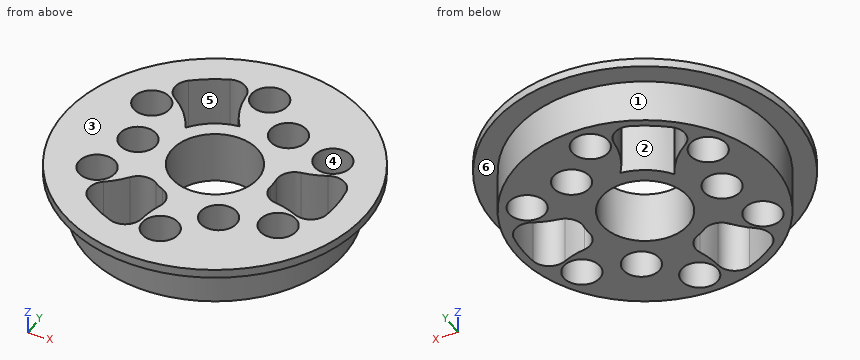
from build123d import *

# Parameters (mm, degrees)
SKETCH_1_R          = 15
SKETCH_1_R_2        = 2.1
EXTRUDE_1_DEPTH     = 6
EXTRUDE_START       = -1
SKETCH_2_R          = 17.5
SKETCH_2_R_2        = 2.1
EXTRUDE_2_DEPTH     = 1
SKETCH_3_R          = 5
CUT_EXTRUDE_1_DEPTH = 10
CUT_EXTRUDE_3_DEPTH = 10
FILLET_1_R          = 2


with BuildPart() as part:
    # 草图1 → 凸台-拉伸1 (new body)
    with BuildSketch(Plane.XY):
        Circle(SKETCH_1_R)
        with Locations((0, 12)):
            Circle(SKETCH_1_R_2, mode=Mode.SUBTRACT)
        with Locations((10.392304845, 6)):
            Circle(SKETCH_1_R_2, mode=Mode.SUBTRACT)
        with Locations((10.392304845, -6)):
            Circle(SKETCH_1_R_2, mode=Mode.SUBTRACT)
        with Locations((0, -12)):
            Circle(SKETCH_1_R_2, mode=Mode.SUBTRACT)
        with Locations((-10.392304845, -6)):
            Circle(SKETCH_1_R_2, mode=Mode.SUBTRACT)
        with Locations((-10.392304845, 6)):
            Circle(SKETCH_1_R_2, mode=Mode.SUBTRACT)
        with Locations((4.425, 7.664324823)):
            Circle(SKETCH_1_R_2, mode=Mode.SUBTRACT)
        with Locations((4.419693866, -7.655134331)):
            Circle(SKETCH_1_R_2, mode=Mode.SUBTRACT)
        with Locations((-8.844693866, 0.009190493)):
            Circle(SKETCH_1_R_2, mode=Mode.SUBTRACT)
    extrude(amount=EXTRUDE_1_DEPTH)

    # 草图2 → 凸台-拉伸2 (add)
    with BuildSketch(Plane.XY.offset(6).offset(EXTRUDE_START)):
        Circle(SKETCH_2_R)
        with Locations((-8.844693866, 0.009190493)):
            Circle(SKETCH_2_R_2, mode=Mode.SUBTRACT)
        with Locations((-10.392304845, -6)):
            Circle(SKETCH_2_R_2, mode=Mode.SUBTRACT)
        with Locations((0, -12)):
            Circle(SKETCH_2_R_2, mode=Mode.SUBTRACT)
        with Locations((4.419693866, -7.655134331)):
            Circle(SKETCH_2_R_2, mode=Mode.SUBTRACT)
        with Locations((10.392304845, -6)):
            Circle(SKETCH_2_R_2, mode=Mode.SUBTRACT)
        with Locations((10.392304845, 6)):
            Circle(SKETCH_2_R_2, mode=Mode.SUBTRACT)
        with Locations((4.425, 7.664324823)):
            Circle(SKETCH_2_R_2, mode=Mode.SUBTRACT)
        with Locations((0, 12)):
            Circle(SKETCH_2_R_2, mode=Mode.SUBTRACT)
        with Locations((-10.392304845, 6)):
            Circle(SKETCH_2_R_2, mode=Mode.SUBTRACT)
    extrude(amount=EXTRUDE_2_DEPTH)

    # 草图3 → 切除-拉伸1 (cut)
    with BuildSketch(Plane.XY.offset(6)):
        Circle(SKETCH_3_R)
    extrude(amount=-CUT_EXTRUDE_1_DEPTH, mode=Mode.SUBTRACT)

    # 草图4 → 切除-拉伸3 (cut)
    with BuildSketch(Plane(origin=(0, 0, 0), x_dir=(-1, 0, 0), z_dir=(0, 0, -1))):
        with BuildLine():
            ThreePointArc((5.465336879, 3.961387736), (7.679309109, 7.001766097), (10.89964539, 8.94470404))
            ThreePointArc((10.89964539, 8.94470404), (7.05, 12.210958193), (2.296518233, 13.91172182))
            ThreePointArc((2.296518233, 13.91172182), (2.224052757, 10.151359821), (0.697993974, 6.713814446))
            ThreePointArc((0.697993974, 6.713814446), (3.375, 5.845671476), (5.465336879, 3.961387736))
        make_face()
        with BuildLine():
            ThreePointArc((2.296518233, -13.91172182), (7.05, -12.210958193), (10.89964539, -8.94470404))
            ThreePointArc((10.89964539, -8.94470404), (7.679309109, -7.001766097), (5.465336879, -3.961387736))
            ThreePointArc((5.465336879, -3.961387736), (3.375, -5.845671476), (0.697993974, -6.713814446))
            ThreePointArc((0.697993974, -6.713814446), (2.224052757, -10.151359821), (2.296518233, -13.91172182))
        make_face()
        with BuildLine():
            ThreePointArc((-6.163330853, 2.75242671), (-9.903361866, 3.149593723), (-13.196163623, 4.96701778))
            ThreePointArc((-13.196163623, 4.96701778), (-14.1, 0), (-13.196163623, -4.96701778))
            ThreePointArc((-13.196163623, -4.96701778), (-9.903361866, -3.149593723), (-6.163330853, -2.75242671))
            ThreePointArc((-6.163330853, -2.75242671), (-6.75, 0), (-6.163330853, 2.75242671))
        make_face()
    extrude(amount=-CUT_EXTRUDE_3_DEPTH, mode=Mode.SUBTRACT)

    # 圆角1
    fillet_1_edges = [part.edges().sort_by_distance(p)[0] for p in [
        (-10.89964539, 8.94470404, 3),
        (-2.296518233, 13.91172182, 3),
        (-2.296518233, -13.91172182, 3),
        (-0.697993974, -6.713814446, 3),
        (-5.465336879, -3.961387736, 3),
        (-10.89964539, -8.94470404, 3),
        (6.163330853, -2.75242671, 3),
        (13.196163623, -4.96701778, 3),
        (13.196163623, 4.96701778, 3),
        (6.163330853, 2.75242671, 3),
    ]]
    fillet(fillet_1_edges, radius=FILLET_1_R)


solid = part.part
Work out the finished part from the listing and answer in its coordinate system (mm). Face numbers are marked on the shaded views. A direction names the side the tool comes from. Round coordinates to 2 decimals unless told otherwise and drop trailing zeros. Order: outer loops, then holes, each group sorted by start corner. A loop starts at its lowest first (then second) coordinate and runs counter-clockwise, first axis right, second up. Notation, with made-up numbers: M 12,41.25 L 53,41.25 A11 cw 53,52.25 Z; hole C 36,86.25 d1. An arc over 180 degrees is marked long. Put each result on its own line as item: value. Start each with the question number.
Q1. Section B-B, the plane y = 6 is taken. Write down the section's boundary in (x, z).
Q2. Flat-ended cylindrical pins translate along their axes: pin 1 (4 mm diameter, centred on x = 0, y = 12, fed in from -Z); pin 2 (1 mm diameter, centred on x = -2, z = 3, fed in from -Y); pin 3 (1.5 mm diameter, centred on x = 11, z = 3, fed in from +Y). Find the tip coordinate at first contact, or state that the pin passes through.
Q3. Straight lines are drawn through the part: L1, parallel to Y at x = 0, z = 1.95; L2, parallel to Y at x = -11, z = 4; L3, parallel to X at y = 1.5, z = 3.25. For each, find the intervals that lie inside material, in ascending order. Write a range as [from, to].
Q4. A tool of negligible diameter and unlimited length cuts with its end or side. For the marked faces 5 and 6, from which of +Z, -Z, +X, -X, +Y, -Y can it reach the whole face along a straight path? Write none if from no direction.
Q5. Section D-D, the plane y = -12 is taken. Give the number of separate pieces and of enclosed holes in the cut face, and give its area (3 significant figures).
Q6. For a pull along Y with two mould halves and no side action, classify the marked faces 1, 2, 3 and 4 as pulls with the +Y half, pulls with the -Y half, needs draft (parallel to the pull), parting line crosses it, or undercut.
Q7. Section C-C, the plane x = -12 is taken. Write down the section's boundary in (y, z).
Q8. Section A-A, the plane x = 0 is taken. Write down the section's boundary in (y, z), and give its area (3 significant figures).
Findings below:
1. outline: M -16.44,5 L -13.75,5 L -13.75,0 L -12.49,0 L -12.49,6 L -16.44,6 Z; M -8.29,0 L -6.73,0 L -6.73,6 L -8.29,6 Z; M -3.09,0 L 3.14,0 L 3.14,6 L -3.09,6 Z; M 5.71,0 L 8.29,0 L 8.29,6 L 5.71,6 Z; M 12.49,0 L 13.75,0 L 13.75,5 L 16.44,5 L 16.44,6 L 12.49,6 Z
2. pin 1: passes through
2. pin 2: stops at y = -14.92
2. pin 3: stops at y = 10.95
3. L1: y = [-15, -14.1], [-9.9, -5], [5, 9.9], [14.1, 15]
3. L2: y = [-10.2, -8.01], [-3.99, 3.99], [8.01, 10.2]
3. L3: x = [-14.92, -10.32], [-7.37, -4.77], [4.77, 6.83], [14.02, 14.92]
4. face 5: +Z, -Z
4. face 6: -Z
5. separate pieces: 3
5. enclosed holes: 0
5. area: 61.2 mm^2
6. face 1: parting line crosses it
6. face 2: undercut
6. face 3: needs draft
6. face 4: undercut
7. outline: M -12.74,5 L -9,5 L -9,0 L -7.35,0 L -7.35,6 L -12.74,6 Z; M -4.65,0 L 4.65,0 L 4.65,6 L -4.65,6 Z; M 7.35,0 L 9,0 L 9,5 L 12.74,5 L 12.74,6 L 7.35,6 Z
8. outline: M -17.5,5 L -15,5 L -15,0 L -14.1,0 L -14.1,6 L -17.5,6 Z; M -9.9,0 L -5,0 L -5,6 L -9.9,6 Z; M 5,0 L 9.9,0 L 9.9,6 L 5,6 Z; M 14.1,0 L 15,0 L 15,5 L 17.5,5 L 17.5,6 L 14.1,6 Z
8. area: 74.6 mm^2
